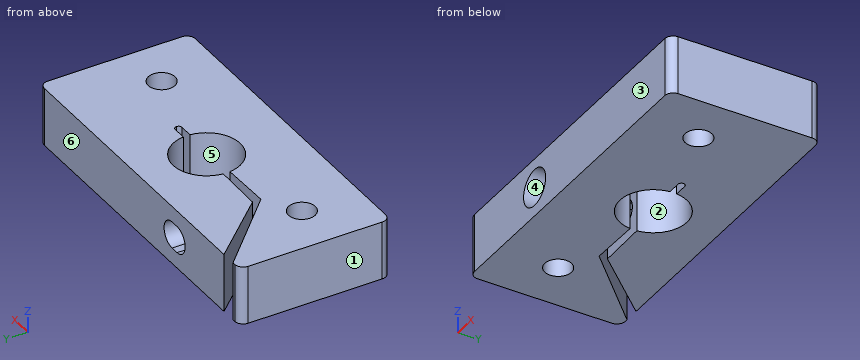
from build123d import *

# Parameters (mm, degrees)
BOSS_EXTRUDE1_DEPTH      = 3.5
BOSS_EXTRUDE1_DEPTH_BACK = 3.5
SKETCH1_R                = 1.6
CUT_EXTRUDE1_REACH       = 29.134
SKETCH3_R                = 1.6
SKETCH3_3_R              = 2.2
SKETCH3_3_R_2            = 1.6
CUT_EXTRUDE2_DEPTH       = 6
CUT_EXTRUDE3_REACH       = 29.134
FILLET1_R                = 1
FILLET2_R                = 0.4


with BuildPart() as part:
    # Sketch1 → Boss-Extrude1 (new, two sides: drawn at the far end of the back side and taken through both)
    with BuildSketch(Plane.XY.offset(-BOSS_EXTRUDE1_DEPTH_BACK)):
        with BuildLine():
            Line((-20, 8), (-18.64966284, 8))
            Line((-18.64966284, 8), (-10, -0.5))
            Line((-10, -0.5), (-3.979949748, -0.4))
            ThreePointArc((-3.979949748, -0.4), (0, -4), (3.979949748, -0.4))
            Line((3.979949748, -0.4), (6, -0.4))
            Line((6, -0.4), (6, 0.4))
            Line((6, 0.4), (3.979949748, 0.4))
            ThreePointArc((3.979949748, 0.4), (0, 4), (-3.979949748, 0.4))
            Line((-3.979949748, 0.4), (-10, 0.5))
            Line((-10, 0.5), (-16.848441102, 8))
            Line((-16.848441102, 8), (20, 8))
            Line((20, 8), (20, -10))
            Line((20, -10), (-20, -10))
            Line((-20, -10), (-20, 8))
        make_face()
        with Locations((-14, -3)):
            Circle(SKETCH1_R, mode=Mode.SUBTRACT)
        with Locations(Location((14, -3, 0), (0, 0, 180))):
            Circle(SKETCH1_R, mode=Mode.SUBTRACT)
    extrude(amount=BOSS_EXTRUDE1_DEPTH + BOSS_EXTRUDE1_DEPTH_BACK)

    # Cut-Extrude1: up to this plane
    cut_extrude1_end = Plane(origin=(-10, -0.5, -3.5), z_dir=(-0.016608865731892127, 0.9998620632762801, 0))
    # Sketch3 → Cut-Extrude1 (cut, up to the surface)
    with BuildSketch(Plane.XZ.offset(10), mode=Mode.PRIVATE) as cut_extrude1_sk1:
        with Locations(Location((-6.989974874, 0, 0), (0, 0, 270))):
            Circle(SKETCH3_R)
    cut_extrude1_tool1 = split(extrude(cut_extrude1_sk1.sketch, amount=-CUT_EXTRUDE1_REACH, mode=Mode.PRIVATE), bisect_by=cut_extrude1_end, keep=Keep.BOTH, mode=Mode.PRIVATE)
    add(cut_extrude1_tool1.solids().sort_by_distance((-6.989975, -10, 0))[0], mode=Mode.SUBTRACT)

    # Sketch3<3> → Cut-Extrude2 (cut)
    with BuildSketch(Plane.XZ.offset(10)):
        with Locations(Location((-6.989974874, 0, 0), (0, 0, 270))):
            Circle(SKETCH3_3_R)
        with Locations(Location((-6.989974874, 0, 0), (0, 0, 270))):
            Circle(SKETCH3_3_R_2, mode=Mode.SUBTRACT)
    extrude(amount=-CUT_EXTRUDE2_DEPTH, mode=Mode.SUBTRACT)

    # Cut-Extrude3: up to this plane
    cut_extrude3_end = Plane(origin=(-10, 0.5, -3.5), z_dir=(-0.016608865731892127, -0.9998620632762801, 0))
    # Sketch4 → Cut-Extrude3 (cut, up to the surface)
    with BuildSketch(Plane(origin=(0, 8, 0), x_dir=(1, 0, 0), z_dir=(0, 1, 0)), mode=Mode.PRIVATE) as cut_extrude3_sk1:
        with BuildLine():
            Line((-7.489974874, 1.6), (-6.489974874, 1.6))
            ThreePointArc((-6.489974874, 1.6), (-4.889974874, 0), (-6.489974874, -1.6))
            Line((-6.489974874, -1.6), (-7.489974874, -1.6))
            ThreePointArc((-7.489974874, -1.6), (-9.089974874, 0), (-7.489974874, 1.6))
        make_face()
    cut_extrude3_tool1 = split(extrude(cut_extrude3_sk1.sketch, amount=-CUT_EXTRUDE3_REACH, mode=Mode.PRIVATE), bisect_by=cut_extrude3_end, keep=Keep.BOTH, mode=Mode.PRIVATE)
    add(cut_extrude3_tool1.solids().sort_by_distance((-6.989975, 8, 0))[0], mode=Mode.SUBTRACT)

    # Fillet1
    fillet1_edges = [part.edges().sort_by_distance(p)[0] for p in [
        (20, 8, 0),
        (20, -10, 0),
        (-20, -10, 0),
        (-20, 8, 0),
    ]]
    fillet(fillet1_edges, radius=FILLET1_R)

    # Fillet2
    fillet2_edges = [part.edges().sort_by_distance(p)[0] for p in [
        (6, -0.4, 0),
        (6, 0.4, 0),
    ]]
    fillet(fillet2_edges, radius=FILLET2_R - 0.0001)  # a hair under: the kernel refuses the full size


solid = part.part
Source: CAD feature listing. Evaluate the final solid. Frame: model axes, mm. Face numbers are marked on the shaded views. A direction names the side the tool comes from. Round coordinates to 2 decimals unless told otherwise and drop trailing zeros. Order: outer loops, then holes, each group sorted by start corner. A loop starts at its lowest first (then second) coordinate and runs counter-clockwise, first axis right, second up. Notation, with made-up numbers: (-23, -33) -> (-14, -33) arc R26 ccw to (-14, -1) -> close; hole circle Ø10 at (53.25, 19). An arc over 180 degrees is marked (long way). Answer as CSV lines item,"result".
Item 1: Section C-C, the plane x = 14. Return loops of the section in (y, z).
A:
outline,"(-10, -3.5) -> (-4.6, -3.5) -> (-4.6, 3.5) -> (-10, 3.5) -> close; (-1.4, -3.5) -> (8, -3.5) -> (8, 3.5) -> (-1.4, 3.5) -> close"
Item 2: Section A-A, the plane z = 0. Count the separate pieces of the cut face and the enclosed holes in it, plus the area to 3 significant figures.
A:
separate pieces,"3"
enclosed holes,"2"
area,"565 mm²"
Item 3: Section D-D, the plane y = -3.5. Return loops of the section in (x, z).
A:
outline,"(-20, -3.5) -> (-15.52, -3.5) -> (-15.52, 3.5) -> (-20, 3.5) -> close; (-12.48, -3.5) -> (-1.94, -3.5) -> (-1.94, 3.5) -> (-12.48, 3.5) -> close; (1.94, -3.5) -> (12.48, -3.5) -> (12.48, 3.5) -> (1.94, 3.5) -> close; (15.52, -3.5) -> (20, -3.5) -> (20, 3.5) -> (15.52, 3.5) -> close; hole circle Ø3.2 at (-6.99, 0)"
Item 4: Pull-direction query (Y, two-part tool) for the marked faces 1, 2 and 3; classes: pulls with the +Y half, pulls with the -Y half, needs draft (parallel to the pull), parting line crosses it, or undercut.
A:
face 1,"needs draft"
face 2,"undercut"
face 3,"pulls with the -Y half"
Item 5: Line query: L1, parallel to Y at x = 14, z = 1.25; L2, parallel to X at y = -3.5, z = -2.5; L3, parallel to X at y = -2.75, z = 0. Output: solid intervals per line, ascending.
A:
L1,"-10 to -4.6, -1.4 to 8"
L2,"-20 to -15.52, -12.48 to -1.94, 1.94 to 12.48, 15.52 to 20"
L3,"-20 to -15.58, -12.42 to -8.59, -5.39 to -2.9, 2.9 to 12.42, 15.58 to 20"
Item 6: Reachability of the marked faces 4, 5 and 6 from +Z, -Z, +X, -X, +Y, -Y: full face, straight path, thin tool, end or side. Return the list, or none.
A:
face 4,"-Y"
face 5,"+Z, -Z"
face 6,"+Z, -Z, +X, -X, +Y"
Item 7: Section B-B, the plane y = 2.5. Return loops of the section in (x, z).
A:
outline,"(-20, -3.5) -> (-13.05, -3.5) -> (-13.05, 3.5) -> (-20, 3.5) -> close; (-11.83, -3.5) -> (-3.12, -3.5) -> (-3.12, 3.5) -> (-11.83, 3.5) -> close; (3.12, -3.5) -> (20, -3.5) -> (20, 3.5) -> (3.12, 3.5) -> close; hole (-7.49, -1.6) -> (-6.49, -1.6) arc R1.6 ccw to (-6.49, 1.6) -> (-7.49, 1.6) arc R1.6 ccw to start"
